Read the model definition and answer for the solid it produces. Units are mm, in the model's axes. Round coordinates to 2 decimals unless told otherwise and drop trailing zeros. Order: outer loops, then holes, each group sorted by start corner. A loop starts at its lowest first (then second) coordinate and runs counter-clockwise, first axis right, second up.
from build123d import *

# Parameters (mm, degrees)
BOSS_EXTRUDE1_DEPTH     = 6.35
CUT_EXTRUDE1_DEPTH      = 280.056311342
CUT_EXTRUDE1_DEPTH_BACK = 280.056311342
SKETCH2_R               = 0.635


with BuildPart() as part:
    # Sketch1 → Boss-Extrude1 (new body)
    with BuildSketch(Plane.XY):
        Polygon((0, 0), (20.32, 0), (20.32, 12.7), (274.32, 12.7), (274.32, 38.1), (20.32, 38.1), (20.32, 50.8), (0, 50.8), align=None)
    extrude(amount=BOSS_EXTRUDE1_DEPTH)

    # Sketch2 → Cut-Extrude1 (cut, two sides: drawn at the far end of the back side and taken through both)
    with BuildSketch(Plane.XY.offset(6.35).offset(-CUT_EXTRUDE1_DEPTH_BACK)):
        with Locations((10.16, 43.688)):
            Circle(SKETCH2_R)
        with Locations((10.16, 25.4)):
            Circle(SKETCH2_R)
        with Locations((10.16, 7.112)):
            Circle(SKETCH2_R)
    extrude(amount=CUT_EXTRUDE1_DEPTH + CUT_EXTRUDE1_DEPTH_BACK, mode=Mode.SUBTRACT)


solid = part.part
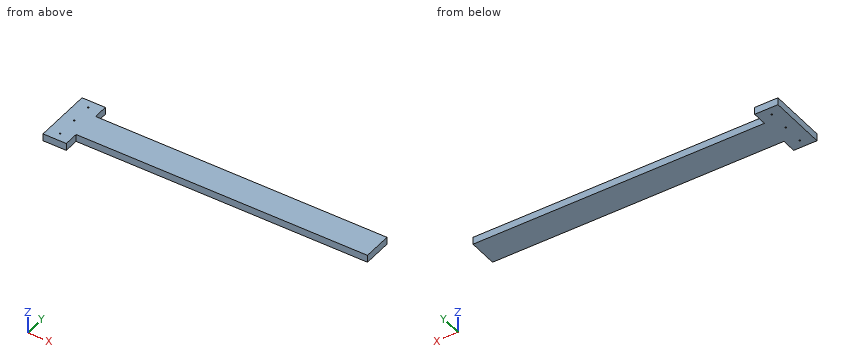
Q1. Flat-ended cylindrical pins translate along their axes: pin 1 (0.8 mm diameter, centred on x = 10.16, y = 43.688, fed in from +Z); pin 2 (3 mm diameter, centred on x = 186, z = 3, fed in from -Y); pin 3 (1.5 mm diameter, centred on x = 10.16, y = 25.4, fed in from +Z); pin 4 (1.9 mm diameter, centred on y = 7, z = 2, fed in from +X). Find the tip coordinate at first contact, or state that the pin passes through.
Outcome:
pin 1: passes through
pin 2: stops at y = 12.7
pin 3: stops at z = 6.35
pin 4: stops at x = 20.32
Q2. A cutting plane is placed at B-B, the plane x = 172. Give the vertices of the cut face in (y, z), plus the area to 3 significant figures.
Outcome:
outline: (12.7, 0) - (38.1, 0) - (38.1, 6.35) - (12.7, 6.35) - close
area: 161 mm2
Q3. Straight lines are drawn through the part: probe 1 along Y at (x, z) = (10.16, 2.5) (3 decimals); probe 2 along X at (y, z) = (25.4, 4) (3 decimals); probe 3 along Y at (x, z) = (100.5, 0.5). For each, find the intervals that lie inside material, in ascending order.
Outcome:
probe 1: y = 0 to 6.477, 7.747 to 24.765, 26.035 to 43.053, 44.323 to 50.8
probe 2: x = 0 to 9.525, 10.795 to 274.32
probe 3: y = 12.7 to 38.1
Q4. A cutting plane is placed at C-C, the plane y = 47.5. Give the vertices of the cut face in (x, z), plus the area to 3 significant figures.
Outcome:
outline: (0, 0) - (20.32, 0) - (20.32, 6.35) - (0, 6.35) - close
area: 129 mm2
Q5. A cutting plane is placed at A-A, the plane z = 2. Give the vertices of the cut face in (x, y) (3 decimals), plus the area to 3 significant figures.
Outcome:
outline: (0, 0) - (20.32, 0) - (20.32, 12.7) - (274.32, 12.7) - (274.32, 38.1) - (20.32, 38.1) - (20.32, 50.8) - (0, 50.8) - close; hole circle Ø1.27 at (10.16, 7.112); hole circle Ø1.27 at (10.16, 25.4); hole circle Ø1.27 at (10.16, 43.688)
area: 7,480 mm2
